Geometry check sheet. Reference: the model listing, model coordinates, mm. Give positions to 0.01 mm unless a question says otherwise; leave off trailing zeros. Write each loop counter-clockwise with the first axis right and the second up, starting at its lowest first coordinate (ties: lowest second). Pieces come first, ordered by that corner, then holes. Notation, with made-up numbers: (22, -6) -> (59, -6) arc R22 ccw to (59, 24) -> close; hole circle Ø9 at (46.25, 40). An arc over 180 degrees is marked (long way). One line per item, written item: value.
from build123d import *

# Parameters (mm, degrees)
SKETCH1_R           = 2
SKETCH1_R_2         = 5
SKETCH1_R_3         = 1.5
BOSS_EXTRUDE1_DEPTH = 4


with BuildPart() as part:
    # Sketch1 → Boss-Extrude1 (new body)
    with BuildSketch(Plane(origin=(0, 0, 0), x_dir=(1, 0, 0), z_dir=(0, 1, 0))):
        with BuildLine():
            ThreePointArc((-31.416051551, 41.741670191), (0, 20.1), (31.416051551, 41.741670191))
            ThreePointArc((31.416051551, 41.741670191), (44.547727215, 44.547727215), (41.741670191, 31.416051551))
            ThreePointArc((41.741670191, 31.416051551), (20.1, 0), (41.741670191, -31.416051551))
            ThreePointArc((41.741670191, -31.416051551), (44.547727215, -44.547727215), (31.416051551, -41.741670191))
            ThreePointArc((31.416051551, -41.741670191), (0, -20.1), (-31.416051551, -41.741670191))
            ThreePointArc((-31.416051551, -41.741670191), (-44.547727215, -44.547727215), (-41.741670191, -31.416051551))
            ThreePointArc((-41.741670191, -31.416051551), (-20.1, 0), (-41.741670191, 31.416051551))
            ThreePointArc((-41.741670191, 31.416051551), (-44.547727215, 44.547727215), (-31.416051551, 41.741670191))
        make_face()
        with Locations(Location((-38.890872965, 38.890872965, 0), (0, 0, 270))):
            Circle(SKETCH1_R, mode=Mode.SUBTRACT)
        with Locations(Location((38.890872965, 38.890872965, 0), (0, 0, 270))):
            Circle(SKETCH1_R, mode=Mode.SUBTRACT)
        with Locations(Location((38.890872965, -38.890872965, 0), (0, 0, 270))):
            Circle(SKETCH1_R, mode=Mode.SUBTRACT)
        with Locations(Location((-38.890872965, -38.890872965, 0), (0, 0, 270))):
            Circle(SKETCH1_R, mode=Mode.SUBTRACT)
        with Locations(Location((0, 0, 0), (0, 0, 270))):
            Circle(SKETCH1_R_2, mode=Mode.SUBTRACT)
        with Locations(Location((20.831365774, 20.831365774, 0), (0, 0, 270))):
            Circle(SKETCH1_R_3, mode=Mode.SUBTRACT)
        with Locations(Location((-20.831365774, -20.831365774, 0), (0, 0, 270))):
            Circle(SKETCH1_R_3, mode=Mode.SUBTRACT)
    extrude(amount=BOSS_EXTRUDE1_DEPTH)


solid = part.part
1) Sectioned sample at C-C on y = 3. Record the cut outline in (x, z), plus the area to 3 significant figures.
Verdict:
outline: (-41.74, -31.42) arc R8 ccw (long way) to (-31.42, -41.74) arc R33.62 cw to (31.42, -41.74) arc R8 ccw (long way) to (41.74, -31.42) arc R33.62 cw to (41.74, 31.42) arc R8 ccw (long way) to (31.42, 41.74) arc R33.62 cw to (-31.42, 41.74) arc R8 ccw (long way) to (-41.74, 31.42) arc R33.62 cw to start; hole circle Ø4 at (-38.89, -38.89); hole circle Ø4 at (-38.89, 38.89); hole circle Ø3 at (-20.83, 20.83); hole circle Ø10 at (0, 0); hole circle Ø3 at (20.83, -20.83); hole circle Ø4 at (38.89, -38.89); hole circle Ø4 at (38.89, 38.89)
area: 3,270 mm^2
2) Depth check by flat-ended pin: pin 1 Ø1.5 at (x, y) = (12, 3) entering from -Z; pin 2 Ø1.5 at (y, z) = (2, -28) entering from -X; pin 3 Ø1 at (y, z) = (2.5, 5) entering from +X. Enter the tip coordinate at first touch or a pass-through.
Verdict:
pin 1: z = -22.61
pin 2: x = -36.29
pin 3: x = 20.55
3) Sectioned sample at B-B on z = 0. Record the cut outline in (x, y).
Verdict:
outline: (-20.1, 0) -> (-5, 0) -> (-5, 4) -> (-20.1, 4) -> close; (5, 0) -> (20.1, 0) -> (20.1, 4) -> (5, 4) -> close
4) Sectioned sample at A-A on x = 0. Record the cut outline in (y, z).
Verdict:
outline: (0, -20.1) -> (4, -20.1) -> (4, -5) -> (0, -5) -> close; (0, 5) -> (4, 5) -> (4, 20.1) -> (0, 20.1) -> close
5) Scan lines: probe 1 along X at (y, z) = (2.6, 0); probe 2 along X at (y, z) = (1.2, 38); probe 3 along X at (y, z) = (3.5, 40). Record each from-to range of solid material in increasing order.
Verdict:
probe 1: -20.1 to -5, 5 to 20.1
probe 2: -46.84 to -40.68, -37.1 to -29.72, 29.72 to 37.1, 40.68 to 46.84
probe 3: -46.81 to -40.56, -37.23 to -30.7, 30.7 to 37.23, 40.56 to 46.81
6) Sectioned sample at D-D on x = -16. Record the cut outline in (y, z).
Verdict:
outline: (0, -24.15) -> (4, -24.15) -> (4, 24.15) -> (0, 24.15) -> close
7) Mould release check, pull along Z, two halves, no side actions. Record for faces 1 (the cylindrical face through (40.874, 1.972, -39.151)), 2 (the flat face through (1, 0, -11)), 3 (the cylindrical face through (-0.568, 1.972, -20.105)), 4 (the cylindrical face through (44.7, 1.97, 44.39)): released by +Z, released by -Z, zero draft, split by the parting line, or undercut.
Verdict:
face 1: undercut
face 2: zero draft
face 3: released by -Z
face 4: undercut
